from build123d import *

# Parameters (mm, degrees)
SKETCH_1_R          = 4
EXTRUDE_1_DEPTH     = 5
CUT_EXTRUDE_1_DEPTH = 2


with BuildPart() as part:
    # 草图1 → 凸台-拉伸1 (new body, symmetric)
    with BuildSketch(Plane(origin=(0, 0, 0), x_dir=(0, 0, -1), z_dir=(1, 0, 0))):
        with BuildLine():
            Line((-40, 8), (40, 8))
            ThreePointArc((40, 8), (48, 0), (40, -8))
            Line((40, -8), (-40, -8))
            ThreePointArc((-40, -8), (-48, 0), (-40, 8))
        make_face()
        with Locations((40, 0)):
            Circle(SKETCH_1_R, mode=Mode.SUBTRACT)
        with Locations((-40, 0)):
            Circle(SKETCH_1_R, mode=Mode.SUBTRACT)
    extrude(amount=EXTRUDE_1_DEPTH, both=True)

    # 草图2 → 切除-拉伸1 (cut)
    with BuildSketch(Plane.ZY.offset(5)):
        with BuildLine():
            Line((-27.5, 5), (27.5, 5))
            ThreePointArc((27.5, 5), (32.5, 0), (27.5, -5))
            Line((27.5, -5), (-27.5, -5))
            ThreePointArc((-27.5, -5), (-32.5, 0), (-27.5, 5))
        make_face()
    cut_extrude_1 = extrude(amount=-CUT_EXTRUDE_1_DEPTH, mode=Mode.SUBTRACT)

    # 镜向1: 切除-拉伸1 across plane
    add(cut_extrude_1.mirror(Plane(origin=(0, 0, 0), x_dir=(0, 0, 1), z_dir=(1, 0, 0))), mode=Mode.SUBTRACT)


solid = part.part
Read the model definition and answer for the solid it produces. Units are mm, in the model's axes. A direction names the side the tool comes from. Give positions to 0.01 mm unless a question says otherwise; leave off trailing zeros. Write each loop counter-clockwise with the first axis right and the second up, starting at its lowest first coordinate (ties: lowest second). Pieces come first, ordered by that corner, then holes. Notation, with made-up numbers: (-13, -22) -> (31, -22) arc R16 cw to (31, -11) -> close; hole circle Ø10 at (41, -32.5). An arc over 180 degrees is marked (long way). Answer as a JSON object with one key per item and string values. Group by question number.
1) Each of these flat-tipped pins is pushed along its axis until it touches: P1, Ø2, axis at y = -3.5, z = 23.5, coming from the -X side; P2, Ø5, axis at x = -0.5, y = 6, coming from the -Z side; P3, Ø5, axis at y = 0, z = 40, coming from the -X side. Where does it stop, or does it pass through?
2) Find section C-C (z = 29.5). Write down the section's boundary in (x, y), and give its area (3 significant figures).
3) Consider L1, parallel to Y at x = -3, z = -40; L2, parallel to Y at x = 4.5, z = 19.5; L3, parallel to Z at x = 0, y = -0.5. Determine where each line is inside the solid, lowest interval first. Write a range as from..to.
4) Find section A-A (x = 1.5). Write down the section's boundary in (y, z).
5) Find section B-B (z = 15.5). Write down the section's boundary in (x, y), and give its area (3 significant figures).
6) The mould has two halves that part along Z. Classify faces 4 (the flat face through (-4, -5, 0)), 5 (the cylindrical face through (0, 0, 48)), 6 (the cylindrical face through (0, 0, -48)): +Z half, -Z half, draft (parallel to the pull), parting line (faces both ways), or undercut.
7) A tool of negligible diameter and unlimited length cuts with its end or side. For faces 1 (the cylindrical face through (-4, -0.1, -32.5)), 2 (the flat face through (-5, 5.4, -0.7)), 3 (the cylindrical face through (4, -0.1, -32.5)), from which of +Z, -Z, +X, -X, +Y, -Y can it reach the whole face along a straight path? Write none if from no direction.
8) Find section D-D (y = 6). Write down the section's boundary in (x, z), and give its area (3 significant figures).
Values follow:
{
 "1": {"P1": "stops at x = -3", "P2": "stops at z = -47.19", "P3": "passes through"},
 "2": {"outline": "(-5, -8) -> (5, -8) -> (5, -4.58) -> (3, -4.58) -> (3, 4.58) -> (5, 4.58) -> (5, 8) -> (-5, 8) -> (-5, 4.58) -> (-3, 4.58) -> (-3, -4.58) -> (-5, -4.58) -> close", "area": "123 mm2"},
 "3": {"L1": "y = -8..-4, 4..8", "L2": "y = -8..-5, 5..8", "L3": "z = -47.98..-43.97, -36.03..36.03, 43.97..47.98"},
 "4": {"outline": "(-8, -40) arc R8 ccw to (8, -40) -> (8, 40) arc R8 ccw to (-8, 40) -> close; hole circle Ø8 at (0, -40); hole circle Ø8 at (0, 40)"},
 "5": {"outline": "(-5, -8) -> (5, -8) -> (5, -5) -> (3, -5) -> (3, 5) -> (5, 5) -> (5, 8) -> (-5, 8) -> (-5, 5) -> (-3, 5) -> (-3, -5) -> (-5, -5) -> close", "area": "120 mm2"},
 "6": {"face 4": "undercut", "face 5": "+Z half", "face 6": "-Z half"},
 "7": {"face 1": "-X", "face 2": "+Z, -Z, -X, +Y, -Y", "face 3": "+X"},
 "8": {"outline": "(-5, -45.29) -> (5, -45.29) -> (5, 45.29) -> (-5, 45.29) -> close", "area": "906 mm2"}
}
